Geometry: final body of the model. Coordinates: model frame, mm. A direction names the side the tool comes from. Give positions to 0.01 mm unless a question says otherwise; leave off trailing zeros. Write each loop counter-clockwise with the first axis right and the second up, starting at its lowest first coordinate (ties: lowest second). Pieces come first, ordered by that corner, then holes. Notation, with made-up numbers: (-21, 54) -> (30, 54) arc R10 cw to (30, 70) -> close; hole circle Ø4 at (88.5, 40). An arc over 180 degrees is marked (long way). Answer in a Markdown table with one row per item. Add a question column.
Item 1: Section query D-D on z = 62.5. Output: boundary loops of the cut face in (x, y).
Item 2: Material intervals for probe 1 along Y at (x, z) = (13.75, 105); probe 2 along Y at (x, z) = (16.4, 10); probe 3 along Z at (x, y) = (11, 4), sorted ascending. Write a range as from..to.
Item 3: Access query for faces 1 (the flat face through (8, 11, 96)), 2 (the flat face through (5.2, 3, 60)), 3 (the flat face through (15.2, 5.8, 10.4)), 4 (the flat face through (4, 15.2, 60)). Directions: +Z, -Z, +X, -X, +Y, -Y. A direction counts if a zero-diameter tool reaches every point of the face in a straight line with its end or side. Return the directions, or none.
Item 4: Draft query along Z for faces 5 (the flat face through (18.2, 7, 60)), 6 (the cylindrical face through (16.7, 6, 9.6)), 7 (the flat face through (13.2, 7.5, 98)). Return one class per face: +Z half, -Z half, draft (parallel to the pull), parting line (faces both ways), or undercut.
Item 5: Section query C-C on x = 3.25. Output: boundary loops of the cut face in (y, z), plus the area to 3 significant figures.
Item 6: Section query B-B on z = 111. Output: boundary loops of the cut face in (x, y), plus the area to 3 significant figures.
Item 7: First-contact query: P1, Ø2, axis at x = 9, y = 8.5, coming from the -Z side; P2, Ø1.8, axis at x = 9, y = 5, coming from the +Z side; P3, Ø5.5, axis at y = 6.5, z = 62.5, coming from the -X side. Flat tips, straight axial feed; report the tip coordinate or a pass-through.
Item 8: Section query A-A on y = 7.6. State how many separate pieces and enclosed holes the cut face has, plus the area to 3 significant figures.
```python
from build123d import *

# Parameters (mm, degrees)
SKETCH_1_W          = 21.2
SKETCH_1_H          = 21.2
SKETCH_1_W_2        = 15.2
SKETCH_1_H_2        = 15.2
EXTRUDE_1_DEPTH     = 121
SKETCH_2_R          = 1.65
CUT_EXTRUDE_1_DEPTH = 30
SKETCH_3_W          = 314.053168424
SKETCH_3_H          = 46.219516436
CUT_EXTRUDE_2_DEPTH = 3
SKETCH_4_W          = 5
SKETCH_4_H          = 15.2
EXTRUDE_1_2_DEPTH   = 10
SKETCH_5_W          = 61
SKETCH_5_H          = 5
EXTRUDE_2_DEPTH     = 10
SKETCH_6_W          = 71
SKETCH_6_H          = 15.2
EXTRUDE_3_DEPTH     = 10
SKETCH_8_W          = 71
SKETCH_8_H          = 5
CUT_EXTRUDE_3_DEPTH = 3
CHAMFER_1_SIZE      = 3
CHAMFER_2_SIZE      = 4


with BuildPart() as part:
    # 草图1 → Extrude 1 (new body)
    with BuildSketch(Plane.XY):
        with Locations((7.6, 7.6)):
            Rectangle(SKETCH_1_W, SKETCH_1_H)
        with Locations((7.6, 7.6)):
            Rectangle(SKETCH_1_W_2, SKETCH_1_H_2, mode=Mode.SUBTRACT)
    extrude(amount=EXTRUDE_1_DEPTH)

    # 草图2 → 切除-拉伸1 (cut)
    with BuildSketch(Plane.ZY.offset(3)):
        with Locations((10, 7.6)):
            Circle(SKETCH_2_R)
        with Locations((111, 7.6)):
            Circle(SKETCH_2_R)
    extrude(amount=-CUT_EXTRUDE_1_DEPTH, mode=Mode.SUBTRACT)

    # 草图3 → 切除-拉伸2 (cut)
    with BuildSketch(Plane.ZY.offset(3)):
        with Locations((151.731232528, 0.202739406)):
            Rectangle(SKETCH_3_W, SKETCH_3_H)
    extrude(amount=-CUT_EXTRUDE_2_DEPTH, mode=Mode.SUBTRACT)

    # 草图4 → Extrude 1 2 (add)
    with BuildSketch(Plane.ZY.offset(-15.2)):
        with Locations((27.5, 7.6)):
            Rectangle(SKETCH_4_W, SKETCH_4_H)
        with Locations((93.5, 7.6)):
            Rectangle(SKETCH_4_W, SKETCH_4_H)
    extrude(amount=EXTRUDE_1_2_DEPTH)

    # 草图5 → 凸台-拉伸2 (add)
    with BuildSketch(Plane.ZY.offset(-15.2)):
        with Locations((60.5, 7.6)):
            Rectangle(SKETCH_5_W, SKETCH_5_H)
    extrude(amount=EXTRUDE_2_DEPTH)

    # 草图6 → 凸台-拉伸3 (add)
    with BuildSketch(Plane.ZY.offset(-15.2)):
        with Locations((60.5, 7.6)):
            Rectangle(SKETCH_6_W, SKETCH_6_H)
    extrude(amount=EXTRUDE_3_DEPTH)

    # 草图8 → 切除-拉伸3 (cut)
    with BuildSketch(Plane.ZY.offset(-5.2)):
        with Locations((60.5, 7.6)):
            Rectangle(SKETCH_8_W, SKETCH_8_H)
    extrude(amount=-CUT_EXTRUDE_3_DEPTH, mode=Mode.SUBTRACT)

    # 倒角1
    chamfer_1_edges = [part.edges().sort_by_distance(p)[0] for p in [
        (8.2, 7.6, 25),
        (8.2, 7.6, 96),
    ]]
    chamfer(chamfer_1_edges, length=CHAMFER_1_SIZE)

    # 倒角2
    chamfer_2_edges = [part.edges().sort_by_distance(p)[0] for p in [
        (15.2, 7.6, 25),
        (15.2, 7.6, 96),
    ]]
    chamfer(chamfer_2_edges, length=CHAMFER_2_SIZE - 0.0001)  # a hair under: the kernel refuses the full size


solid = part.part
```
Findings below:
| question | item | result |
|---|---|---|
| 1 | outline | (0, -3) -> (18.2, -3) -> (18.2, 18.2) -> (0, 18.2) -> (0, 15.2) -> (5.2, 15.2) -> (5.2, 10.1) -> (8.2, 10.1) -> (8.2, 5.1) -> (5.2, 5.1) -> (5.2, 0) -> (0, 0) -> close |
| 2 | probe 1 | y = -3..0, 15.2..18.2 |
| 2 | probe 2 | y = -3..5.95, 9.25..18.2 |
| 2 | probe 3 | z = 25..96 |
| 3 | face 1 | +Z, -X |
| 3 | face 2 | +Z, -Z, -X |
| 3 | face 3 | -Z, -X |
| 3 | face 4 | -X |
| 4 | face 5 | draft |
| 4 | face 6 | undercut |
| 4 | face 7 | +Z half |
| 5 | outline | (-3, 0) -> (0, 0) -> (0, 121) -> (-3, 121) -> close; (15.2, 0) -> (18.2, 0) -> (18.2, 121) -> (15.2, 121) -> close |
| 5 | area | 726 mm^2 |
| 6 | outline | (0, -3) -> (18.2, -3) -> (18.2, 5.95) -> (15.2, 5.95) -> (15.2, 0) -> (0, 0) -> close; (0, 15.2) -> (15.2, 15.2) -> (15.2, 9.25) -> (18.2, 9.25) -> (18.2, 18.2) -> (0, 18.2) -> close |
| 6 | area | 145 mm^2 |
| 7 | P1 | stops at z = 26.2 |
| 7 | P2 | stops at z = 96 |
| 7 | P3 | stops at x = 5.2 |
| 8 | separate pieces | 3 |
| 8 | enclosed holes | 0 |
| 8 | area | 847 mm^2 |
